Check sheet for the modelled part. Datum: model origin and axes. Units: mm. A direction names the side the tool comes from. Round coordinates to 2 decimals unless told otherwise and drop trailing zeros. Write each loop counter-clockwise with the first axis right and the second up, starting at its lowest first coordinate (ties: lowest second). Pieces come first, ordered by that corner, then holes.
Item 1: Tool access check on faces 4 (the flat face through (-950, 451, -696)), 5 (the flat face through (-507, 399, -1000)). Record the directions out of +Z, -Z, +X, -X, +Y, -Y that give a thin tool (end or side, any length) a straight path to the whole face; none if there is none.
Item 2: Go/stop test with a flat-tipped pin: pin 1 Ø10 at (x, z) = (-709.5, -400) entering from +Y. Record where the tip stops, or that it passes through.
Item 3: Release check for a two-part mould opening along X. For faces 1 (the flat face through (-493, 399, 0)), 2 (the flat face through (-1000, 399, -493)), 3 (the flat face through (-350, 451, -223)) record: +X half, -X half, draft (parallel to the pull), parting line (faces both ways), or undercut.
Item 4: Cross-section at B-B on z = -113.5. Enter the section's corners in (x, y).
Item 5: Cross-section at D-D on y = 383. Enter the section's corners in (x, z).
Item 6: Material ranges on line 1 (X direction, y = 432.5, z = -899); line 2 (X direction, y = 428.5, z = -85); line 3 (Z direction, x = -675, y = 472), recorded low to high.
Item 7: Cross-section at C-C on x = -456. Enter the section's corners in (y, z).
Item 8: Cross-section at A-A on x = -730. Enter the section's corners in (y, z).
Autodesk Inventor part; units mm, degrees
ref_plane "YZ Plane" through (0, 0, 0) normal (1, 0, 0) x (0, 1, 0)
ref_plane "XZ Plane" through (0, 0, 0) normal (0, 1, 0) x (-1, 0, 0)
ref_plane "XY Plane" through (0, 0, 0) normal (0, 0, 1) x (1, 0, 0)
sketch "Sketch1" plane through (0, 0, 0) normal (0, 1, 0) x (-1, 0, 0)
  line L0 (0, 0) -> (1000, 0)
  line L1 (1000, 0) -> (1000, -1000)
  line L2 (1000, -1000) -> (0, -1000)
  line L3 (0, -1000) -> (0, 0)
  dimension "d0" = 1000
  dimension "d1" = 1000
  dimension "d2" = 1000
extrude "Extrusion1" add sketch "Sketch1" along normal blind 500
sketch "Sketch2" plane through (0, 500, 0) normal (0, 1, 0) x (1, 0, 0)
  point P0 (0, 0)
sketch "Sketch3" plane through (0, 500, 0) normal (0, 1, 0) x (1, 0, 0)
  point P0 (0, 0)
sketch "Sketch4" plane through (0, 500, 0) normal (0, 1, 0) x (1, 0, 0)
  line L0 (-1000, 0) -> (0, 0)
  line L1 (-50, 50) -> (-50, 200)
  line L2 (-50, 200) -> (-200, 200)
  line L3 (-200, 200) -> (-350, 200)
  line L4 (-350, 200) -> (-350, 50)
  line L5 (-350, 50) -> (-50, 50)
  dimension "d7" = 150
  dimension "d8" = 150
  dimension "d9" = 150
  dimension "d10" = 150
  dimension "d13" = 200
  dimension "d14" = 50
extrude "Extrusion2" cut sketch "Sketch4" against normal blind 100
sketch "Sketch5" plane through (0, 500, 0) normal (0, 1, 0) x (1, 0, 0)
  line L0 (-350, 200) -> (-50, 200)
  line L1 (-350, 200) -> (-350, 400)
  line L2 (-350, 400) -> (-50, 400)
  line L3 (-50, 400) -> (-50, 250)
  line L4 (-50, 250) -> (-200, 250)
  line L5 (-200, 250) -> (-200, 200)
  point P0 (0, 0)
  dimension "d17" = 200
  dimension "d18" = 300
  dimension "d19" = 150
  dimension "d20" = 150
extrude "Extrusion3" cut sketch "Sketch5" against normal blind 100
sketch "Sketch6" plane through (0, 500, 0) normal (0, 1, 0) x (1, 0, 0)
  line L0 (-50, 400) -> (-50, 250)
  line L1 (-50, 400) -> (-50, 900)
  line L2 (-50, 900) -> (-50, 950)
  line L3 (-50, 950) -> (-550, 950)
  line L4 (-550, 950) -> (-550, 800)
  line L5 (-550, 800) -> (-250, 800)
  line L6 (-250, 800) -> (-200, 800)
  line L7 (-200, 800) -> (-200, 400)
  line L8 (-350, 400) -> (-50, 400)
  line L9 (-200, 400) -> (-50, 400)
  point P0 (0, 0)
  dimension "d23" = 500
  dimension "d24" = 50
  dimension "d25" = 500
  dimension "d26" = 150
  dimension "d27" = 300
  dimension "d28" = 50
extrude "Extrusion4" cut sketch "Sketch6" against normal blind 100
sketch "Sketch7" plane through (0, 500, 0) normal (0, 1, 0) x (1, 0, 0)
  line L0 (-250, 800) -> (-250, 500)
  line L1 (-250, 500) -> (-250, 450)
  line L2 (-250, 450) -> (-400, 450)
  line L3 (-400, 450) -> (-400, 50)
  line L4 (-400, 50) -> (-550, 50)
  line L5 (-550, 50) -> (-550, 200)
  line L6 (-550, 200) -> (-550, 400)
  line L7 (-550, 400) -> (-550, 600)
  line L8 (-550, 600) -> (-550, 700)
  line L9 (-550, 700) -> (-400, 700)
  line L10 (-400, 700) -> (-400, 800)
  line L11 (-400, 800) -> (-250, 800)
  point P0 (0, 0)
  point P1 (-200, 800)
  dimension "d32" = 50
  dimension "d33" = 300
  dimension "d34" = 50
  dimension "d35" = 150
  dimension "d36" = 400
  dimension "d37" = 150
  dimension "d38" = 150
  dimension "d39" = 200
  dimension "d40" = 200
  dimension "d41" = 100
  dimension "d42" = 150
  dimension "d43" = 250
extrude "Extrusion5" cut sketch "Sketch7" against normal blind 100
sketch "Sketch8" plane through (0, 500, 0) normal (0, 1, 0) x (1, 0, 0)
  point P0 (0, 0)
sketch "Sketch9" plane through (0, 500, 0) normal (0, 1, 0) x (1, 0, 0)
  point P0 (0, 0)
sketch "Sketch10" plane through (0, 500, 0) normal (0, 1, 0) x (1, 0, 0)
  line L0 (0, 0) -> (0, 1000)
  line L1 (-550, 50) -> (-550, 200)
  line L2 (-550, 50) -> (-550, 700)
  line L3 (-550, 200) -> (-650, 200)
  line L4 (-650, 200) -> (-850, 200)
  line L5 (-850, 200) -> (-900, 200)
  line L6 (-900, 200) -> (-950, 200)
  line L7 (-950, 200) -> (-950, 50)
  line L8 (-950, 50) -> (-550, 50)
  point P0 (-400, 50)
  dimension "d48" = 150
  dimension "d49" = 150
  dimension "d50" = 100
  dimension "d51" = 200
  dimension "d52" = 50
  dimension "d53" = 50
extrude "Extrusion6" cut sketch "Sketch10" against normal blind 100
sketch "Sketch11" plane through (0, 500, 0) normal (0, 1, 0) x (1, 0, 0)
  line L0 (-700, 200) -> (-700, 250)
  line L1 (-700, 250) -> (-600, 250)
  line L2 (-600, 250) -> (-600, 400)
  line L3 (-600, 400) -> (-950, 400)
  line L4 (-950, 400) -> (-950, 200)
  line L5 (-950, 200) -> (-700, 200)
  point P0 (0, 0)
  dimension "d60" = 50
  dimension "d61" = 100
  dimension "d62" = 150
  dimension "d63" = 350
extrude "Extrusion7" cut sketch "Sketch11" against normal blind 100
sketch "Sketch12" plane through (0, 500, 0) normal (0, 1, 0) x (1, 0, 0)
  point P0 (0, 0)
sketch "Sketch13" plane through (0, 500, 0) normal (0, 1, 0) x (1, 0, 0)
  line L0 (0, 0) -> (0, 1000)
  line L1 (-600, 400) -> (-600, 550)
  line L2 (-600, 550) -> (-600, 600)
  line L3 (-950, 600) -> (-950, 450)
  line L4 (-950, 450) -> (-750, 450)
  line L5 (-750, 450) -> (-750, 400)
  line L6 (-750, 400) -> (-600, 400)
  line L7 (-950, 600) -> (-950, 950)
  line L8 (-950, 950) -> (-650, 950)
  line L9 (-650, 950) -> (-600, 950)
  line L10 (-600, 950) -> (-600, 650)
  line L11 (-600, 650) -> (-750, 650)
  line L12 (-750, 650) -> (-750, 700)
  line L13 (-750, 700) -> (-750, 800)
  line L14 (-750, 800) -> (-800, 800)
  line L15 (-800, 800) -> (-800, 600)
  line L16 (-600, 600) -> (-600, 400)
  line L17 (-800, 600) -> (-600, 600)
  dimension "d69" = 150
  dimension "d70" = 50
  dimension "d71" = 350
  dimension "d72" = 150
  dimension "d73" = 200
  dimension "d74" = 350
  dimension "d75" = 300
  dimension "d76" = 50
  dimension "d77" = 300
  dimension "d79" = 50
  dimension "d80" = 100
  dimension "d81" = 50
  dimension "d82" = 90
  dimension "d83" = 600
  dimension "d84" = 750
extrude "Extrusion8" cut sketch "Sketch13" against normal blind 100
sketch "Sketch14" plane through (0, 400, 0) normal (0, 1, 0) x (1, 0, 0)
  circle A0 centre (-882.0732, 213.6869) radius 50
  point P0 (0, 0)
  dimension "d87" = 100
  dimension "d88" = 907.5875
extrude "Extrusion9" cut sketch "Sketch14" against normal blind 500
sketch "Sketch15" plane through (0, 400, 0) normal (0, 1, 0) x (1, 0, 0)
  circle A0 centre (-473.0021, 632.6041) radius 50
  point P0 (0, 0)
  dimension "d91" = 100
  dimension "d92" = 789.8854
extrude "Extrusion10" cut sketch "Sketch15" against normal blind 500
sketch "Sketch16" plane through (0, 0, 0) normal (0, -1, 0) x (1, 0, 0)
  line L0 (0, -1000) -> (0, 0)
  line L1 (0, 0) -> (0, -1000)
  line L2 (0, -1000) -> (-1000, -1000)
  line L3 (-1000, -1000) -> (-1000, 0)
  line L4 (-1000, -1000) -> (-1000, 0)
  line L5 (-1000, 0) -> (0, 0)
  line L6 (-1000, 0) -> (0, 0)
extrude "Extrusion11" cut sketch "Sketch16" against normal blind 300
Response values:
1. face 4: +Y
1. face 5: -Z, +X, -X, +Y, -Y
2. pin 1: stops at y = 400
3. face 1: draft
3. face 2: -X half
3. face 3: undercut
4. outline: (-1000, 300) - (0, 300) - (0, 500) - (-50, 500) - (-50, 400) - (-350, 400) - (-350, 500) - (-400, 500) - (-400, 400) - (-950, 400) - (-950, 500) - (-1000, 500) - close
5. outline: (-1000, -1000) - (0, -1000) - (0, 0) - (-1000, 0) - close; hole circle Ø100 at (-882.07, -213.69); hole circle Ø100 at (-473, -632.6)
6. line 1: x = -1000 to -950, -600 to -550, -50 to 0
6. line 2: x = -1000 to -950, -400 to -350, -50 to 0
6. line 3: z = -1000 to -950, -650 to -600, -250 to -200, -50 to 0
7. outline: (300, -1000) - (500, -1000) - (500, -950) - (400, -950) - (400, -800) - (500, -800) - (500, -700) - (400, -700) - (400, -679.62) - (300, -679.62) - close; (300, -585.58) - (400, -585.58) - (400, -50) - (500, -50) - (500, 0) - (300, 0) - close
8. outline: (300, -1000) - (500, -1000) - (500, -950) - (400, -950) - (400, -650) - (500, -650) - (500, -600) - (400, -600) - (400, -50) - (500, -50) - (500, 0) - (300, 0) - close
